Check sheet for the modelled part. Datum: model origin and axes. Units: mm. A direction names the side the tool comes from. Coordinates: 2 decimals unless noted, no trailing zeros. Write each loop counter-clockwise with the first axis right and the second up, starting at its lowest first coordinate (ties: lowest second). Pieces come first, ordered by that corner, then holes. Notation, with made-up numbers: (77.25, 68.25) -> (82.25, 68.25) arc R32 cw to (82.25, 101.25) -> close; hole circle Ø10 at (13.25, 16). An arc over 180 degrees is marked (long way). Put each result on its own line as item: value.
```python
from build123d import *

# Parameters (mm, degrees)
BOSS_EXTRUDE1_DEPTH  = 10
BOSS_EXTRUDE6_DEPTH  = 41
CUT_EXTRUDE1_REACH   = 81.124
CUT_EXTRUDE2_REACH   = 81.124
BOSS_EXTRUDE9_DEPTH  = 10
CHAMFER3_SIZE        = 10
BOSS_EXTRUDE10_DEPTH = 55.75
CUT_EXTRUDE3_REACH   = 118.716
SKETCH12_R           = 2


with BuildPart() as part:
    # Sketch2 → Boss-Extrude1 (new body)
    with BuildSketch(Plane.XY):
        Polygon((-5, -51.344559606), (-5, -0.20517252), (44.083730464, 1.808954014), (44.083730464, -19.205040291), (14.477900916, -51.344559606), align=None)
    extrude(amount=BOSS_EXTRUDE1_DEPTH)

    # Sketch2<5> → Boss-Extrude6 (add)
    with BuildSketch(Plane.XY):
        Polygon((-5, -51.344559606), (14.477900916, -51.344559606), (14.477900916, -46.344559606), (0, -46.344559606), (0, 0), (-5, -0.20517252), align=None)
    extrude(amount=-BOSS_EXTRUDE6_DEPTH)

    # Sketch6 → Cut-Extrude1 (cut, up to next)
    with BuildSketch(Plane(origin=(0, 0, 0), x_dir=(0, 0, -1), z_dir=(1, 0, 0)), mode=Mode.PRIVATE) as cut_extrude1_sk1:
        with BuildLine():
            Line((31.5, 0), (41, 0))
            Line((41, 0), (41, -24.844559606))
            ThreePointArc((41, -24.844559606), (47.717514421, -41.062074027), (31.5, -34.344559606))
            Line((31.5, -34.344559606), (31.5, 0))
        make_face()
    cut_extrude1_tool1 = extrude(cut_extrude1_sk1.sketch, amount=-CUT_EXTRUDE1_REACH, mode=Mode.PRIVATE) & part.part
    add(cut_extrude1_tool1.solids().sort_by_distance((0, -24.478408, -38.654556))[0], mode=Mode.SUBTRACT)

    # Sketch7 → Cut-Extrude2 (cut, up to next)
    with BuildSketch(Plane(origin=(0, 0, 0), x_dir=(-1, 0, 0), z_dir=(0, 0, -1)), mode=Mode.PRIVATE) as cut_extrude2_sk1:
        Polygon((-39.083730464, -17.253097249), (-16.891496625, -41.344559606), (-5, -41.344559606), (-5, -4.799035286), (-39.083730464, -3.400426311), align=None)
    cut_extrude2_tool1 = extrude(cut_extrude2_sk1.sketch, amount=-CUT_EXTRUDE2_REACH, mode=Mode.PRIVATE) & part.part
    add(cut_extrude2_tool1.solids().sort_by_distance((19.604261, -19.893914, 0))[0], mode=Mode.SUBTRACT)

    # Sketch10 → Boss-Extrude9 (add)
    with BuildSketch(Plane.XY.offset(-29)):
        Polygon((14.477900916, -46.344559606), (0, -46.344559606), (0, 0), (10, 0.41034504), (10, -36.344559606), (14.477900916, -36.344559606), align=None)
    extrude(amount=BOSS_EXTRUDE9_DEPTH)

    # Chamfer3
    chamfer3_edges = [part.edges().sort_by_distance(p)[0] for p in [
        (12.238950458, -36.344559606, -19),
        (10, -17.967107283, -19),
    ]]
    chamfer(chamfer3_edges, length=CHAMFER3_SIZE - 0.0001)  # a hair under: the kernel refuses the full size

    # Sketch11 → Boss-Extrude10 (add)
    with BuildSketch(Plane(origin=(0, 0, -41), x_dir=(-1, 0, 0), z_dir=(0, 0, -1))):
        Polygon((5, -51.344559606), (5, -43.844559606), (0, -43.844559606), (0, -46.344559606), (-14.477900916, -46.344559606), (-14.477900916, -51.344559606), align=None)
    extrude(amount=BOSS_EXTRUDE10_DEPTH)

    # Sketch12 → Cut-Extrude3 (cut, up to next)
    with BuildSketch(Plane(origin=(0, -46.344559606, 0), x_dir=(1, 0, 0), z_dir=(0, 1, 0)), mode=Mode.PRIVATE) as cut_extrude3_sk1:
        with Locations(Location((5, 58.5, 0), (0, 0, 180))):
            Circle(SKETCH12_R)
    cut_extrude3_tool1 = extrude(cut_extrude3_sk1.sketch, amount=-CUT_EXTRUDE3_REACH, mode=Mode.PRIVATE) & part.part
    add(cut_extrude3_tool1.solids().sort_by_distance((5, -46.34456, -58.5))[0], mode=Mode.SUBTRACT)

    # Mirror3: part across plane


with BuildPart() as part_1:
    add(part.part)
    add(part.part.mirror(Plane(origin=(0, 0, -96.75), x_dir=(1, 0, 0), z_dir=(0, 0, -1))))


solid = part_1.part
```
Q1. Cross-section at A-A (z = -135). Record the cut outline in (x, y), plus the area to 3 significant figures.
Recorded:
outline: (-5, -51.34) -> (3, -51.34) -> (3, -46.34) -> (0, -46.34) -> (0, -43.84) -> (-5, -43.84) -> close; (7, -51.34) -> (14.48, -51.34) -> (14.48, -46.34) -> (7, -46.34) -> close
area: 89.9 mm2
Q2. Cross-section at C-C (z = -5). Record the cut outline in (x, y).
Recorded:
outline: (-5, -51.34) -> (14.48, -51.34) -> (14.48, -46.34) -> (0, -46.34) -> (0, 0) -> (-5, -0.21) -> close
Q3. Material ranges on line 1 along Z through (x, y) = (5, -48); line 2 along Z through (x, y) = (12.5, -3); line 3 along Y through (x, z) = (11, -117.5), recorded low to high.
Recorded:
line 1: z = -203.5 to -137, -133 to -60.5, -56.5 to 10
line 2: z = -203.5 to -193.5, 0 to 10
line 3: y = -51.34 to -46.34
Q4. Cross-section at D-D (x = 12). State how many separate pieces and enclosed holes the cut face has, plus the area to 3 significant figures.
Recorded:
separate pieces: 3
enclosed holes: 0
area: 1,370 mm2
Q5. Mould release check, pull along Z, two halves, no side actions. Record for faces 1 (the flat face through (39.084, -10, 5)), 2 (the flat face through (-3, -43.845, -98)): released by +Z, released by -Z, zero draft, split by the parting line, or undercut.
Recorded:
face 1: zero draft
face 2: undercut
Q6. Tool access check on faces 3 (the flat face through (14.478, -47, -97)), 4 (the flat face through (5, -23, 5)), 5 (the flat face through (7, -46.345, -9)). Record the directions out of +Z, -Z, +X, -X, +Y, -Y that give a thin tool (end or side, any length) a straight path to the whole face; none if there is none.
Recorded:
face 3: +X, +Y, -Y
face 4: +Z
face 5: +X, +Y
Q7. Depth check by flat-ended pin: P1, Ø5, axis at x = 8, y = -14.5, coming from the -Z side; P2, Ø16, axis at x = 5, z = -11, coming from the +Y side; P3, Ø2.5, axis at x = 5, z = -58.5, coming from the +Y side (3 decimals); P4, Ø11, axis at x = 11.5, z = 7.5, coming from the +Y side. Enter the tip coordinate at first touch or a pass-through.
Recorded:
P1: stops at z = -169
P2: stops at y = 0
P3: passes through
P4: stops at y = 0.7
Q8. Cross-section at B-B (x = 35). Record the cut outline in (y, z).
Recorded:
outline: (-29.07, -203.5) -> (-21.69, -203.5) -> (-21.69, -193.5) -> (-29.07, -193.5) -> close; (-29.07, 0) -> (-21.69, 0) -> (-21.69, 10) -> (-29.07, 10) -> close; (-3.57, -203.5) -> (1.44, -203.5) -> (1.44, -193.5) -> (-3.57, -193.5) -> close; (-3.57, 0) -> (1.44, 0) -> (1.44, 10) -> (-3.57, 10) -> close
